For this review, take the finished solid that the model builds, in its own axes (mm). Face numbers are marked on the shaded views. A direction names the side the tool comes from. Give positions to 0.01 mm unless a question says otherwise; leave off trailing zeros. Loops run counter-clockwise (first coordinate to the right, second up) from the corner with the lowest first, then second, coordinate; pieces in that order, holes last. Notation, with made-up numbers: (29, 21.25) - (77, 21.25) arc R26 cw to (77, 55.25) - close; hole circle Ø7 at (11.25, -3). An arc over 180 degrees is marked (long way). Answer in a Markdown table with one row per item.
```python
from build123d import *

# Parameters (mm, degrees)
CROQUIS1_W              = 25
CROQUIS1_H              = 25
SALIENTE_EXTRUIR1_DEPTH = 200
REDONDEO1_R             = 10
REDONDEO2_R             = 10
REDONDEO3_R             = 5
REDONDEO4_R             = 5
CROQUIS2_R              = 11
CROQUIS2_R_2            = 8.5
CORTAR_EXTRUIR1_DEPTH   = 6
CORTAR_EXTRUIR2_START   = -6
CROQUIS3_R              = 8.5
CORTAR_EXTRUIR2_DEPTH   = 6
CROQUIS9_R              = 5.1
CROQUIS9_R_2            = 6
CORTAR_EXTRUIR6_DEPTH   = 30
CROQUIS13_W             = 1
CROQUIS13_H             = 5
CORTAR_EXTRUIR8_DEPTH   = 1
SALIENTE_EXTRUIR3_START = 1
CROQUIS14_R             = 11
CROQUIS14_R_2           = 5.1
SALIENTE_EXTRUIR3_DEPTH = 1
CROQUIS15_R             = 1.5
CORTAR_EXTRUIR9_DEPTH   = 16
CORTAR_EXTRUIR10_DEPTH  = 11
CORTAR_EXTRUIR12_REACH  = 205.101
CROQUIS18_W             = 1
CROQUIS18_H             = 1
CROQUIS19_W             = 17
CROQUIS19_H             = 145
CORTAR_EXTRUIR13_DEPTH  = 10
CROQUIS20_W             = 17
CROQUIS20_H             = 145
CORTAR_EXTRUIR14_DEPTH  = 10
CROQUIS12_R             = 2.25
CORTAR_EXTRUIR7_DEPTH   = 204.100960116


with BuildPart() as part:
    # Croquis1 → Saliente-Extruir1 (new body)
    with BuildSketch(Plane(origin=(0, 0, 0), x_dir=(1, 0, 0), z_dir=(0, 1, 0))):
        with Locations((12.5, 12.5)):
            Rectangle(CROQUIS1_W, CROQUIS1_H)
    extrude(amount=SALIENTE_EXTRUIR1_DEPTH)

    # Redondeo1
    redondeo1_edges = [part.edges().sort_by_distance(p)[0] for p in [
        (12.5, 0, -25),
    ]]
    fillet(redondeo1_edges, radius=REDONDEO1_R)

    # Redondeo2
    redondeo2_edges = [part.edges().sort_by_distance(p)[0] for p in [
        (12.5, 0, 0),
    ]]
    fillet(redondeo2_edges, radius=REDONDEO2_R)

    # Redondeo3
    redondeo3_edges = [part.edges().sort_by_distance(p)[0] for p in [
        (12.5, 200, 0),
    ]]
    fillet(redondeo3_edges, radius=REDONDEO3_R)

    # Redondeo4
    redondeo4_edges = [part.edges().sort_by_distance(p)[0] for p in [
        (12.5, 200, -25),
    ]]
    fillet(redondeo4_edges, radius=REDONDEO4_R)

    # Croquis2 → Cortar-Extruir1 (cut)
    with BuildSketch(Plane(origin=(25, 0, 0), x_dir=(0, 0, -1), z_dir=(1, 0, 0))):
        with Locations((12.5, 187.5)):
            Circle(CROQUIS2_R)
        with Locations(Location((12.5, 12.5, 0), (0, 0, 180))):
            Circle(CROQUIS2_R_2)
    extrude(amount=-CORTAR_EXTRUIR1_DEPTH, mode=Mode.SUBTRACT)

    # Croquis3 → Cortar-Extruir2 (cut)
    with BuildSketch(Plane.ZY.offset(CORTAR_EXTRUIR2_START)):
        with Locations((-12.5, 12.5)):
            Circle(CROQUIS3_R)
        with Locations(Location((-12.5, 187.5, 0), (0, 0, 180))):
            Circle(CROQUIS3_R)
    extrude(amount=CORTAR_EXTRUIR2_DEPTH, mode=Mode.SUBTRACT)

    # Croquis9 → Cortar-Extruir6 (cut)
    with BuildSketch(Plane(origin=(19, 0, 0), x_dir=(0, 0, -1), z_dir=(1, 0, 0))):
        with Locations((12.5, 187.5)):
            Circle(CROQUIS9_R)
        with Locations((12.5, 12.5)):
            Circle(CROQUIS9_R_2)
    extrude(amount=-CORTAR_EXTRUIR6_DEPTH, mode=Mode.SUBTRACT)

    # Croquis13 → Cortar-Extruir8 (cut)
    with BuildSketch(Plane(origin=(0, 0, -25), x_dir=(-1, 0, 0), z_dir=(0, 0, -1))):
        with Locations((-12.5, 187.04733642)):
            Rectangle(CROQUIS13_W, CROQUIS13_H)
    extrude(amount=-CORTAR_EXTRUIR8_DEPTH, mode=Mode.SUBTRACT)

    # Croquis14 → Saliente-Extruir3 (add)
    with BuildSketch(Plane(origin=(19, 0, 0), x_dir=(0, 0, -1), z_dir=(1, 0, 0)).offset(SALIENTE_EXTRUIR3_START)):
        with Locations((12.5, 187.5)):
            Circle(CROQUIS14_R)
        with Locations((12.5, 187.5)):
            Circle(CROQUIS14_R_2, mode=Mode.SUBTRACT)
    extrude(amount=-SALIENTE_EXTRUIR3_DEPTH)

    # Croquis15 → Cortar-Extruir9 (cut)
    with BuildSketch(Plane(origin=(20, 0, 0), x_dir=(0, 0, -1), z_dir=(1, 0, 0))):
        with Locations((17.980077554, 182.019922446)):
            Circle(CROQUIS15_R)
        with Locations((7.019922446, 182.019922446)):
            Circle(CROQUIS15_R)
        with Locations((7.019922446, 192.980077554)):
            Circle(CROQUIS15_R)
        with Locations((17.980077554, 192.980077554)):
            Circle(CROQUIS15_R)
    extrude(amount=-CORTAR_EXTRUIR9_DEPTH, mode=Mode.SUBTRACT)

    # Croquis16 → Cortar-Extruir10 (cut)
    with BuildSketch(Plane.ZY):
        Polygon((-14.829996635, 192.251844396), (-15.774368679, 195.344011075), (-18.924449599, 196.072244234), (-21.130158474, 193.708310713), (-20.185786429, 190.616144033), (-17.035705509, 189.887910875), align=None)
        Polygon((-17.251844396, 185.170003365), (-20.344011075, 184.225631321), (-21.072244234, 181.075550401), (-18.708310713, 178.869841526), (-15.616144033, 179.814213571), (-14.887910875, 182.964294491), align=None)
        Polygon((-7.748155604, 189.829996635), (-4.655988925, 190.774368679), (-3.927755766, 193.924449599), (-6.291689287, 196.130158474), (-9.383855967, 195.185786429), (-10.112089125, 192.035705509), align=None)
        Polygon((-10.170003365, 182.748155604), (-9.225631321, 179.655988925), (-6.075550401, 178.927755766), (-3.869841526, 181.291689287), (-4.814213571, 184.383855967), (-7.964294491, 185.112089125), align=None)
    extrude(amount=-CORTAR_EXTRUIR10_DEPTH, mode=Mode.SUBTRACT)

    # Cortar-Extruir12: up to this face of the body (flat: up to its plane)
    cortar_extruir12_end = Plane(part.part.faces().sort_by_distance((0, 99.909973265, -12.5))[0])
    # Croquis18 → Cortar-Extruir12 (cut, up to the picked face)
    with BuildSketch(Plane(origin=(25, 0, 0), x_dir=(0, 0, -1), z_dir=(1, 0, 0)), mode=Mode.PRIVATE) as cortar_extruir12_sk1:
        with Locations((24.5, 187.5)):
            Rectangle(CROQUIS18_W, CROQUIS18_H)
    cortar_extruir12_tool1 = split(extrude(cortar_extruir12_sk1.sketch, amount=-CORTAR_EXTRUIR12_REACH, mode=Mode.PRIVATE), bisect_by=cortar_extruir12_end, keep=Keep.BOTH, mode=Mode.PRIVATE)
    # Croquis18 → Cortar-Extruir12 (cut, up to the picked face)
    with BuildSketch(Plane(origin=(25, 0, 0), x_dir=(0, 0, -1), z_dir=(1, 0, 0)), mode=Mode.PRIVATE) as cortar_extruir12_sk2:
        with Locations((24.5, 12.5)):
            Rectangle(CROQUIS18_W, CROQUIS18_H)
    cortar_extruir12_tool2 = split(extrude(cortar_extruir12_sk2.sketch, amount=-CORTAR_EXTRUIR12_REACH, mode=Mode.PRIVATE), bisect_by=cortar_extruir12_end, keep=Keep.BOTH, mode=Mode.PRIVATE)
    add(cortar_extruir12_tool1.solids().sort_by(Axis((25, 187.5, -24.5), (-1, 0, 0)))[0], mode=Mode.SUBTRACT)
    add(cortar_extruir12_tool2.solids().sort_by(Axis((25, 12.5, -24.5), (-1, 0, 0)))[0], mode=Mode.SUBTRACT)

    # Croquis19 → Cortar-Extruir13 (cut)
    with BuildSketch(Plane(origin=(25, 0, 0), x_dir=(0, 0, -1), z_dir=(1, 0, 0))):
        with Locations((12.5, 97.5)):
            Rectangle(CROQUIS19_W, CROQUIS19_H)
    extrude(amount=-CORTAR_EXTRUIR13_DEPTH, mode=Mode.SUBTRACT)

    # Croquis20 → Cortar-Extruir14 (cut)
    with BuildSketch(Plane.ZY):
        with Locations((-12.5, 97.5)):
            Rectangle(CROQUIS20_W, CROQUIS20_H)
    extrude(amount=-CORTAR_EXTRUIR14_DEPTH, mode=Mode.SUBTRACT)

    # Croquis12 → Cortar-Extruir7 (cut, through all)
    with BuildSketch(Plane(origin=(0, 0, -25), x_dir=(-1, 0, 0), z_dir=(0, 0, -1))):
        with Locations((-13.6, 187.5)):
            Circle(CROQUIS12_R)
    extrude(amount=-CORTAR_EXTRUIR7_DEPTH, mode=Mode.SUBTRACT)


solid = part.part
```
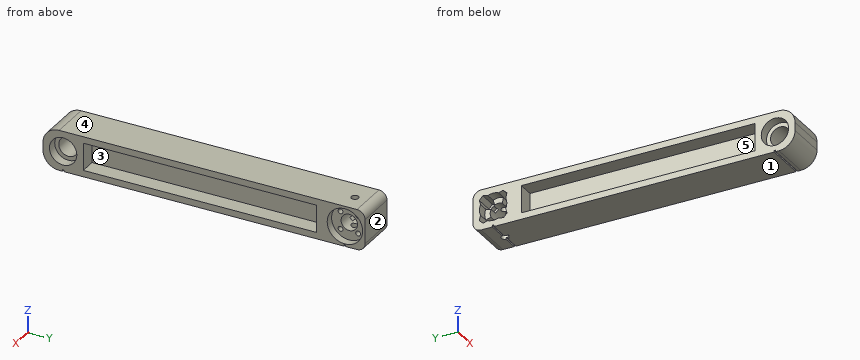
1. We need section A-A, the plane y = 45.5. Give the boundary of the cut face in (x, z), and give its area (3 significant figures).
Values:
| item | result |
|---|---|
| outline | (0, -25) - (25, -25) - (25, -21) - (15, -21) - (15, -4) - (25, -4) - (25, 0) - (0, 0) - (0, -4) - (10, -4) - (10, -21) - (0, -21) - close |
| area | 285 mm^2 |
2. Clearance check with flat-ended pins moving along their axes: pin 1 (5 mm diameter, centred on y = 182.02, z = -17.98, fed in from -X); pin 2 (0.5 mm diameter, centred on x = 12.5, z = -24.5, fed in from -Y); pin 3 (0.5 mm diameter, centred on x = 4.5, z = -24.5, fed in from +Y); pin 4 (10 mm diameter, centred on y = 12.5, z = -12.5, fed in from +X). State where each tip first meets the part, or that it passes through.
Values:
| item | result |
|---|---|
| pin 1 | stops at x = 11 |
| pin 2 | stops at y = 6.2 |
| pin 3 | stops at y = 197.63 |
| pin 4 | passes through |
3. We need section B-B, the plane z = -12.5. Count the separate pieces of the cut face and the enclosed holes in it, and give its area (3 significant figures).
Values:
| item | result |
|---|---|
| separate pieces | 3 |
| enclosed holes | 0 |
| area | 1,390 mm^2 |
4. Wall thickness on line 1 (Y direction, x = 16, z = -12.5); line 2 (Z direction, x = 7, y = 55.5); line 3 (Y direction, x = 9, z = -8.25): over which ranges is each line inside the solid? List them lowest first. Write a range as [from, to].
Values:
| item | result |
|---|---|
| line 1 | y = [0, 6.5], [18.5, 25], [170, 182.4], [192.6, 200] |
| line 2 | z = [-25, -21], [-4, 0] |
| line 3 | y = [0.15, 8.26], [16.74, 25], [170, 179.43], [195.53, 200] |
5. For the marked faces 4 and 5, list the 3-axis set-ups (+Z, -Z, +X, -X, +Y, -Y) from which the entire face can be reached by the end or side of a thin tool; tool diameter is ignored.
Values:
| item | result |
|---|---|
| face 4 | +Z, +X, -X, +Y, -Y |
| face 5 | -X |
6. Mouldability with a two-part tool opening along Y and no side actions: class the marked faces 1, 2 and 3 as released by +Y, released by -Y, zero draft, split by the parting line, or undercut.
Values:
| item | result |
|---|---|
| face 1 | zero draft |
| face 2 | released by +Y |
| face 3 | undercut |
